from build123d import *

# Parameters (mm, degrees)
F0_W     = 57.90056
F0_H     = 40
F1_DEPTH = 1.8
F2_W     = 1.8
F2_H     = 40
F3_DEPTH = 40
F4_R     = 1.875
F5_DEPTH = 9.2


with BuildPart() as f1:
    # F0 (on Top) → F1 (new body)
    with BuildSketch(Plane.XY):
        Rectangle(F0_W, F0_H)
    extrude(amount=F1_DEPTH)

    # F2 (on face) → F3 (join)
    with BuildSketch(Plane.XY.offset(1.8)):
        with Locations((-28.05028, 0)):
            Rectangle(F2_W, F2_H)
    extrude(amount=F3_DEPTH)

    # F4 (on face) → F5 (cut)
    with BuildSketch(Plane(origin=(-28.95028, 0, 0), x_dir=(0, -1, 0), z_dir=(-1, 0, 0))):
        with Locations((14.657458, 36.595527)):
            Circle(F4_R)
        with Locations((-12.731545, 6.108502)):
            Circle(F4_R)
    extrude(amount=-F5_DEPTH, mode=Mode.SUBTRACT)


solid = f1.part
Design review of the part built by this model. Coordinates are the model's own, in mm. A direction names the side the tool comes from. Coordinates: 2 decimals unless noted, no trailing zeros. Loops run counter-clockwise (first coordinate to the right, second up) from the corner with the lowest first, then second, coordinate; pieces in that order, holes last. Notation, with made-up numbers: (-25.75, -26) -> (-10.75, -26) arc R6 cw to (-10.75, -22) -> close; hole circle Ø8 at (-23.5, 32.25). An arc over 180 degrees is marked (long way). Use a Markdown table: item, result. Add a question column.
Item 1: Machinability: for faces 1 (the flat face through (1, 0, 1.8)), 2 (the flat face through (-28, 0, 41.8)), which of the approach directions +Z, -Z, +X, -X, +Y, -Y give a long, thin tool a straight path to every point of the face, cutting with its end or side? Answer none if there is none.
Item 2: The part is to be moulded in two halves that separate along Y. For faces 3 (the flat face through (-13, 20, 1)), 4 (the cylindrical face through (-28.063, -14.413, 38.455)), 5 (the cylindrical face through (-28.063, 14.605, 6.191)), 6 (the flat face through (-13, -20, 1)), say which applies: +Y half, -Y half, draft (parallel to the pull), parting line (faces both ways), or undercut.
Item 3: We need section B-B, the plane z = 27. Write out the cut boundary in (x, y), and give its area (3 significant figures).
Item 4: We need section C-C, the plane x = 21.5. Write out the cut boundary in (y, z), and give its area (3 significant figures).
Item 5: We need section A-A, the plane y = -11. Write out the cut boundary in (x, z), and give its area (3 significant figures).
Item 6: Clearance check with flat-ended pins moving along their axes: P1, Ø5, axis at x = 20, y = 10, coming from the +Z side; P2, Ø12, axis at y = -4, z = 19, coming from the +X side. State where each tip first meets the part, or that it passes through.
Item 7: Wall thickness on L1, parallel to Z at x = -12, y = 16; L2, parallel to X at y = -11, z = 28: over which ranges is each line inside the solid? List them lowest first. Write a range as from..to.
Numbers:
| question | item | result |
|---|---|---|
| 1 | face 1 | +Z, +X, +Y, -Y |
| 1 | face 2 | +Z, +X, -X, +Y, -Y |
| 2 | face 3 | +Y half |
| 2 | face 4 | undercut |
| 2 | face 5 | undercut |
| 2 | face 6 | -Y half |
| 3 | outline | (-28.95, -20) -> (-27.15, -20) -> (-27.15, 20) -> (-28.95, 20) -> close |
| 3 | area | 72.0 mm^2 |
| 4 | outline | (-20, 0) -> (20, 0) -> (20, 1.8) -> (-20, 1.8) -> close |
| 4 | area | 72.0 mm^2 |
| 5 | outline | (-28.95, 0) -> (28.95, 0) -> (28.95, 1.8) -> (-27.15, 1.8) -> (-27.15, 41.8) -> (-28.95, 41.8) -> close |
| 5 | area | 176 mm^2 |
| 6 | P1 | stops at z = 1.8 |
| 6 | P2 | stops at x = -27.15 |
| 7 | L1 | z = 0..1.8 |
| 7 | L2 | x = -28.95..-27.15 |
